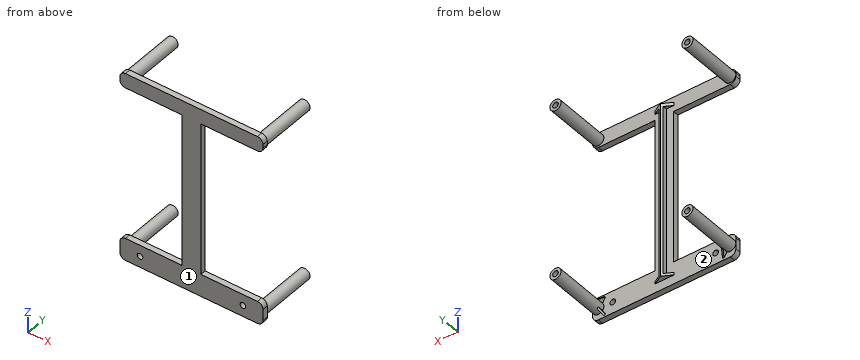
```python
from build123d import *

# Parameters (mm, degrees)
SKETCH_1_W          = 70.5
SKETCH_1_H          = 12
SKETCH_1_R          = 1.5
EXTRUDE_2_DEPTH     = 4
SKETCH_3_W          = 10
SKETCH_3_H          = 82
EXTRUDE_3_DEPTH     = 3
EXTRUDE_4_DEPTH     = 3
SKETCH_5_W          = 70.5
SKETCH_5_H          = 12.216564443
CUT_EXTRUDE_1_DEPTH = 1
SKETCH_6_R          = 3
EXTRUDE_5_DEPTH     = 30
SKETCH_7_W          = 12
SKETCH_7_H          = 3
EXTRUDE_6_DEPTH     = 3
SKETCH_8_W          = 12
SKETCH_8_H          = 3
EXTRUDE_7_DEPTH     = 3
SKETCH_10_W         = 7.85
SKETCH_10_H         = 3
EXTRUDE_8_DEPTH     = 3
SKETCH_11_W         = 7.85
SKETCH_11_H         = 3
EXTRUDE_9_DEPTH     = 3
FILLET_1_R          = 3
EXTRUDE_10_DEPTH    = 3
SKETCH_26_R         = 1.5
CUT_EXTRUDE_2_DEPTH = 30
SKETCH_28_R         = 1.5
CUT_EXTRUDE_3_DEPTH = 30
SKETCH_30_R         = 1.5
CUT_EXTRUDE_4_DEPTH = 30
SKETCH_29_R         = 1.5
CUT_EXTRUDE_5_DEPTH = 30


with BuildPart() as part:
    # 草图1 → 凸台-拉伸2 (new body)
    with BuildSketch(Plane(origin=(0, 0, 0), x_dir=(1, 0, 0), z_dir=(0, 1, 0))):
        with Locations((-4.632001312, -3.115886014)):
            Rectangle(SKETCH_1_W, SKETCH_1_H)
        with Locations((-32.132001312, -3.115886014)):
            Circle(SKETCH_1_R, mode=Mode.SUBTRACT)
        with Locations((22.867998688, -3.115886014)):
            Circle(SKETCH_1_R, mode=Mode.SUBTRACT)
    extrude(amount=EXTRUDE_2_DEPTH)

    # 草图3 → 凸台-拉伸3 (add)
    with BuildSketch(Plane.XZ):
        with Locations((-4.632001312, 50.115886014)):
            Rectangle(SKETCH_3_W, SKETCH_3_H)
    extrude(amount=-EXTRUDE_3_DEPTH)

    # 草图4 → 凸台-拉伸4 (add)
    with BuildSketch(Plane(origin=(0, 3, 0), x_dir=(1, 0, 0), z_dir=(0, 1, 0))):
        Polygon((-4.632001312, -91.115886014), (-39.882001312, -91.115886014), (-39.882001312, -98.965886014), (30.617998688, -98.965886014), (30.617998688, -91.115886014), align=None)
    extrude(amount=-EXTRUDE_4_DEPTH)

    # 草图5 → 切除-拉伸1 (cut)
    with BuildSketch(Plane(origin=(0, 4, 0), x_dir=(1, 0, 0), z_dir=(0, 1, 0))):
        with Locations((-4.632001312, -3.224168236)):
            Rectangle(SKETCH_5_W, SKETCH_5_H)
    extrude(amount=-CUT_EXTRUDE_1_DEPTH, mode=Mode.SUBTRACT)

    # 草图6 → 凸台-拉伸5 (add)
    with BuildSketch(Plane(origin=(0, 3, 0), x_dir=(1, 0, 0), z_dir=(0, 1, 0))):
        with Locations((30.617998688, -3.115886014)):
            Circle(SKETCH_6_R)
        with Locations((-39.882001312, -3.115886014)):
            Circle(SKETCH_6_R)
        with Locations((30.617998688, -95.040886014)):
            Circle(SKETCH_6_R)
        with Locations((-39.882001312, -95.040886014)):
            Circle(SKETCH_6_R)
    extrude(amount=EXTRUDE_5_DEPTH)

    # 草图7 → 凸台-拉伸6 (add)
    with BuildSketch(Plane(origin=(30.617998688, 0, 0), x_dir=(0, 0, -1), z_dir=(1, 0, 0))):
        with Locations((-3.115886014, 1.5)):
            Rectangle(SKETCH_7_W, SKETCH_7_H)
    extrude(amount=EXTRUDE_6_DEPTH)

    # 草图8 → 凸台-拉伸7 (add)
    with BuildSketch(Plane.ZY.offset(39.882001312)):
        with Locations((3.115886014, 1.5)):
            Rectangle(SKETCH_8_W, SKETCH_8_H)
    extrude(amount=EXTRUDE_7_DEPTH)

    # 草图10 → 凸台-拉伸8 (add)
    with BuildSketch(Plane(origin=(30.617998688, 0, 0), x_dir=(0, 0, -1), z_dir=(1, 0, 0))):
        with Locations((-95.040886014, 1.5)):
            Rectangle(SKETCH_10_W, SKETCH_10_H)
    extrude(amount=EXTRUDE_8_DEPTH)

    # 草图11 → 凸台-拉伸9 (add)
    with BuildSketch(Plane.ZY.offset(39.882001312)):
        with Locations((95.040886014, 1.5)):
            Rectangle(SKETCH_11_W, SKETCH_11_H)
    extrude(amount=EXTRUDE_9_DEPTH)

    # 圆角1
    fillet_1_edges = [part.edges().sort_by_distance(p)[0] for p in [
        (-42.882001312, 1.5, 9.115886014),
        (-42.882001312, 1.5, -2.884113986),
        (33.617998688, 1.5, -2.884113986),
        (33.617998688, 1.5, 9.115886014),
        (33.617998688, 1.5, 91.115886014),
        (33.617998688, 1.5, 98.965886014),
        (-42.882001312, 1.5, 91.115886014),
        (-42.882001312, 1.5, 98.965886014),
    ]]
    fillet(fillet_1_edges, radius=FILLET_1_R)

    # 草图12 → 凸台-拉伸10 (add)
    with BuildSketch(Plane(origin=(0, 3, 0), x_dir=(1, 0, 0), z_dir=(0, 1, 0))):
        Polygon((-39.882001312, -3.115886014), (-36.574447776, 1.890119339), (-35.74011355, 1.338860417), (-38.729397599, -3.185441847), (-36.305878929, -8.036388905), (-37.200450273, -8.483314078), align=None)
        Polygon((30.617998688, -3.115886014), (27.617998688, 2.080266408), (26.800231701, 1.50471697), (29.487170484, -3.115886014), (26.765595108, -7.789153997), (27.617998688, -8.312038437), align=None)
        Polygon((-9.960523859, -3.236448921), (-5.714518795, -3.236448921), (-5.714518795, -94.31838866), (-9.960523859, -94.31838866), (-9.960523859, -96.014577306), (0.358950446, -96.014577306), (0.358950446, -94.31838866), (-3.561614819, -94.31838866), (-3.561614819, -3.236448921), (0.358950446, -3.236448921), (0.358950446, -1.92078538), (0, -1.92078538), (-9.960523859, -1.92078538), align=None)
    extrude(amount=EXTRUDE_10_DEPTH)

    # 切除-扫描1: sweep along a path in 草图14
    with BuildLine(Plane(origin=(-10.245146765, 0, 15.506101105), x_dir=(-0.834334226, 0, -0.551258923), z_dir=(0.551258923, 0, -0.834334226))) as sweep_1_path:
        Line((30.557258713, 3), (31.557258713, 3))
    # 草图13 → 切除-扫描1 (sweep, cut)
    with BuildSketch(Plane(origin=(-25.494966785, 0, -16.844961522), x_dir=(0.551258923, 0, -0.834334226), z_dir=(0.834334226, 0, 0.551258923))):
        Polygon((-21.756572303, 6), (-18.584999427, 3), (-18.584999427, 6), align=None)
    sweep(path=sweep_1_path.line, mode=Mode.SUBTRACT)

    # 切除-扫描2: sweep along a path in 草图16
    with BuildLine(Plane(origin=(-4.038812737, 0, -8.084141049), x_dir=(0.894571344, 0, -0.446925173), z_dir=(0.446925173, 0, 0.894571344))) as sweep_2_path:
        Line((-37.069863413, 3), (-36.069863413, 3))
    # 草图15 → 切除-扫描2 (sweep, cut)
    with BuildSketch(Plane(origin=(-33.161637535, 0, 16.567455127), x_dir=(0.446925173, 0, 0.894571344), z_dir=(-0.894571344, 0, 0.446925173))):
        Polygon((-12.036888006, 6), (-9.036888006, 3), (-9.036888006, 6), align=None)
    sweep(path=sweep_2_path.line, mode=Mode.SUBTRACT)

    # 切除-扫描3: sweep along a path in 草图18
    with BuildLine(Plane(origin=(8.169550431, 0, 11.607671187), x_dir=(-0.817766986, 0, 0.575549439), z_dir=(-0.575549439, 0, -0.817766986))) as sweep_3_path:
        Line((-23.782383716, 3), (-22.782383716, 3))
    # 草图17 → 切除-扫描3 (sweep, cut)
    with BuildSketch(Plane(origin=(21.614280794, 0, -12.479010835), x_dir=(-0.5, 0, -0.866025404), z_dir=(0.866025404, 0, -0.5))):
        Polygon((-15.007435787, 6), (-12.007435787, 3), (-12.007435787, 6), align=None)
    sweep(path=sweep_3_path.line, mode=Mode.SUBTRACT)

    # 切除-扫描4: sweep along a path in 草图20
    with BuildLine(Plane(origin=(3.846238842, 0, -6.270119175), x_dir=(0.852403579, 0, 0.52288444), z_dir=(-0.52288444, 0, 0.852403579))) as sweep_4_path:
        Line((27.887916501, 3), (26.887916501, 3))
    # 草图19 → 切除-扫描4 (sweep, cut)
    with BuildSketch(Plane(origin=(24.312717238, 0, 14.036953842), x_dir=(0.5, 0, -0.866025404), z_dir=(0.866025404, 0, 0.5))):
        Polygon((9.6105629, 6), (6.6105629, 3), (6.6105629, 6), align=None)
    sweep(path=sweep_4_path.line, mode=Mode.SUBTRACT)

    # 切除-扫描8: sweep along a path in 草图25
    with BuildLine(Plane(origin=(0, 3, 0), x_dir=(1, 0, 0), z_dir=(0, 1, 0))) as sweep_8_path:
        Line((-4.800786706, -1.92078538), (-4.632001312, -98.965886014))
    # 草图24 → 切除-扫描8 (sweep, cut)
    with BuildSketch(Plane(origin=(0, 0, 1.92078538), x_dir=(-1, 0, 0), z_dir=(0, 0, -1))):
        Polygon((-0.358950446, 3), (4.800786706, 5.789897824), (9.960523859, 3), (10.109613681, 3), (10.681927492, 3), (10.681927492, 6), (10.109613681, 6), (-0.358950446, 6), align=None)
    sweep(path=sweep_8_path.line, mode=Mode.SUBTRACT)

    # 草图26 → 切除-拉伸2 (cut)
    with BuildSketch(Plane(origin=(0, 33, 0), x_dir=(1, 0, 0), z_dir=(0, 1, 0))):
        with Locations((-39.882001312, -95.040886014)):
            Circle(SKETCH_26_R)
    extrude(amount=-CUT_EXTRUDE_2_DEPTH, mode=Mode.SUBTRACT)

    # 草图28 → 切除-拉伸3 (cut)
    with BuildSketch(Plane(origin=(0, 33, 0), x_dir=(1, 0, 0), z_dir=(0, 1, 0))):
        with Locations((30.617998688, -95.040886014)):
            Circle(SKETCH_28_R)
    extrude(amount=-CUT_EXTRUDE_3_DEPTH, mode=Mode.SUBTRACT)

    # 草图30 → 切除-拉伸4 (cut)
    with BuildSketch(Plane(origin=(0, 33, 0), x_dir=(1, 0, 0), z_dir=(0, 1, 0))):
        with Locations((30.617998688, -3.115886014)):
            Circle(SKETCH_30_R)
    extrude(amount=-CUT_EXTRUDE_4_DEPTH, mode=Mode.SUBTRACT)

    # 草图29 → 切除-拉伸5 (cut)
    with BuildSketch(Plane(origin=(0, 33, 0), x_dir=(1, 0, 0), z_dir=(0, 1, 0))):
        with Locations((-39.882001312, -3.115886014)):
            Circle(SKETCH_29_R)
    extrude(amount=-CUT_EXTRUDE_5_DEPTH, mode=Mode.SUBTRACT)


solid = part.part
```
The listing builds one solid part. Answer for the finished solid, in the listing's coordinates (mm). Face numbers are marked on the shaded views. A direction names the side the tool comes from. Round coordinates to 2 decimals unless told otherwise and drop trailing zeros. Write each loop counter-clockwise with the first axis right and the second up, starting at its lowest first coordinate (ties: lowest second). Pieces come first, ordered by that corner, then holes. Notation, with made-up numbers: (17.5, 27) -> (75.5, 27) arc R18 cw to (75.5, 46) -> close; hole circle Ø4 at (46, 9). An arc over 180 degrees is marked (long way). Write item = value, one per line.
1) Section A-A on x = -18.5 is taken. Write down the section's boundary in (y, z), plus the area to 4 significant figures.
Check values:
outline = (0, -2.88) -> (3, -2.88) -> (3, 9.12) -> (0, 9.12) -> close; (0, 91.12) -> (3, 91.12) -> (3, 98.97) -> (0, 98.97) -> close
area = 59.55 mm²
2) Given pin 1 (0.8 mm diameter, centred on x = -5, y = 4.5, fed in from -Z); pin 2 (5 mm diameter, centred on x = -33.5, y = 22, fed in from -Z); pin 3 (1.4 mm diameter, centred on x = -3, y = 4.5, fed in from +Z); pin 4 (1.8 mm diameter, centred on x = -39.88, z = 95.04, fed in from +Y), each flat-ended and moving along its own axis, determine where each tip first touches the part or whether it passes through.
Check values:
pin_1 = 1.92
pin_2 = through
pin_3 = 96.01
pin_4 = 3
3) Section D-D on x = -32 is taken. Write down the section's boundary in (y, z).
Check values:
outline = (0, -2.88) -> (3, -2.88) -> (3, 1.62) -> (0, 1.62) -> close; (0, 4.61) -> (3, 4.61) -> (3, 9.12) -> (0, 9.12) -> close; (0, 91.12) -> (3, 91.12) -> (3, 98.97) -> (0, 98.97) -> close
4) Straight lines are drawn through the part: line 1 along Y through (x, z) = (-7, 53); line 2 along Z through (x, y) = (30, 11); line 3 along X through (y, z) = (10, 3.5). For each, find the intervals that lie inside material, in ascending order. Write a range as [from, to].
Check values:
line_1 = [0, 3]
line_2 = [0.18, 1.75], [4.48, 6.05], [92.11, 93.67], [96.41, 97.98]
line_3 = [-42.86, -41.33], [-38.43, -36.91], [27.64, 29.17], [32.07, 33.59]
5) Section C-C on z = 39 is taken. Write down the section's boundary in (x, y).
Check values:
outline = (-9.63, 0) -> (0.37, 0) -> (0.37, 3) -> (-3.56, 3) -> (-3.56, 5.15) -> (-4.74, 5.79) -> (-5.71, 5.26) -> (-5.71, 3) -> (-9.63, 3) -> close
6) Section B-B on y = 30 is taken. Write down the section's boundary in (x, z), plus the area to 3 significant figures.
Check values:
outline = circle Ø6 at (-39.88, 3.12); circle Ø6 at (-39.88, 95.04); circle Ø6 at (30.62, 3.12); circle Ø6 at (30.62, 95.04); hole circle Ø3 at (-39.88, 3.12); hole circle Ø3 at (-39.88, 95.04); hole circle Ø3 at (30.62, 3.12); hole circle Ø3 at (30.62, 95.04)
area = 84.8 mm²
7) Which of the six approach directions +Z, -Z, +X, -X, +Y, -Y give full straight-line access (tool end or side, diameter ignored) to the marked faces 1 and 2?
Check values:
face_1 = +Z, -Z, +X, -X, -Y
face_2 = +Y
